from build123d import *
from build123d.topology import SkipClean

# Parameters (mm, degrees)
SKETCH1_W           = 100
SKETCH1_H           = 100
BOSS_EXTRUDE1_DEPTH = 100
CUT_EXTRUDE1_DEPTH  = 50
CIRPATTERN1_START   = -50
CIRPATTERN1_DEPTH   = 100
CIRPATTERN1_2_DEPTH = 50
SKETCH3_R           = 12.5
CUT_EXTRUDE2_DEPTH  = 22


with BuildPart() as part:
    # Sketch1 → Boss-Extrude1 (new body)
    with BuildSketch(Plane(origin=(0, 0, 0), x_dir=(1, 0, 0), z_dir=(0, 1, 0))):
        Rectangle(SKETCH1_W, SKETCH1_H)
    extrude(amount=BOSS_EXTRUDE1_DEPTH)

    # Sketch2 → Cut-Extrude1 (cut)
    with BuildSketch(Plane.ZY.offset(50)):
        with BuildLine():
            Line((0, 17.495781671), (-23.033292242, 50))
            ThreePointArc((-23.033292242, 50), (-11.516646121, 61.516646121), (0, 50))
            ThreePointArc((0, 50), (11.516646121, 61.516646121), (23.033292242, 50))
            Line((23.033292242, 50), (0, 17.495781671))
        make_face()
    extrude(amount=-CUT_EXTRUDE1_DEPTH, mode=Mode.SUBTRACT)

    # CirPattern1: read off the stored shape, not the designer's step
    # CirPattern1 outline → CirPattern1 (cut)
    with SkipClean():  # the faces are left unmerged after this step: merging them gives an invalid solid
        with BuildSketch(Plane.XY.offset(CIRPATTERN1_START)):
            with BuildLine():
                Line((-23.033292242, 50), (0, 17.495781671))
                Line((0, 17.495781671), (23.033292242, 50))
                ThreePointArc((23.033292242, 50), (11.516646121, 61.516646121), (0, 50))
                ThreePointArc((0, 50), (-11.516646121, 61.516646121), (-23.033292242, 50))
            make_face()
        extrude(amount=CIRPATTERN1_DEPTH, mode=Mode.SUBTRACT)

    # CirPattern1 2 outline → CirPattern1 2 (cut)
    with SkipClean():  # the faces are left unmerged after this step: merging them gives an invalid solid
        with BuildSketch(Plane.YZ):
            with BuildLine():
                Line((17.495781671, 0), (50, -23.033292242))
                ThreePointArc((50, -23.033292242), (61.516646121, -11.516646121), (50, 0))
                ThreePointArc((50, 0), (61.516646121, 11.516646121), (50, 23.033292242))
                Line((50, 23.033292242), (17.495781671, 0))
            make_face()
        extrude(amount=CIRPATTERN1_2_DEPTH, mode=Mode.SUBTRACT)

    # Sketch3 → Cut-Extrude2 (cut)
    with SkipClean():  # the faces are left unmerged after this step: merging them gives an invalid solid
        with BuildSketch(Plane(origin=(0, 100, 0), x_dir=(1, 0, 0), z_dir=(0, 1, 0))):
            with Locations(Location((0, 0, 0), (0, 0, 270))):
                Circle(SKETCH3_R)
        extrude(amount=-CUT_EXTRUDE2_DEPTH, mode=Mode.SUBTRACT)


solid = part.part
Source: CAD feature listing. Evaluate the final solid. Frame: model axes, mm. A direction names the side the tool comes from. Give positions to 0.01 mm unless a question says otherwise; leave off trailing zeros. Write each loop counter-clockwise with the first axis right and the second up, starting at its lowest first coordinate (ties: lowest second). Pieces come first, ordered by that corner, then holes. Notation, with made-up numbers: (-6.75, 54.5) -> (11.25, 54.5) arc R22 cw to (11.25, 74.5) -> close; hole circle Ø2 at (1.5, 9.5). An arc over 180 degrees is marked (long way). Write item = value, one per line.
Q1. Cut plane C-C on x = 7. Return loops of the section in (y, z).
Here are the results:
outline = (0, -50) -> (27.37, -50) -> (27.37, -7) -> (17.5, 0) -> (27.37, 7) -> (27.37, 50) -> (0, 50) -> close; (60.59, -50) -> (100, -50) -> (100, -10.36) -> (78, -10.36) -> (78, 10.36) -> (100, 10.36) -> (100, 50) -> (60.59, 50) -> (60.59, 16.03) arc R11.52 cw to (60.59, 7) -> (60.59, -7) arc R11.52 cw to (60.59, -16.03) -> close
Q2. Reachability of faces 1 (the face through (-35.304, 61.514, 11.263)), 2 (the face through (11.601, 61.516, -0.054)), 3 (the face through (-12, 100, -12)) from +Z, -Z, +X, -X, +Y, -Y: full face, straight path, thin tool, end or side. Return the list, or none.
Here are the results:
face_1 = +X, -X
face_2 = +Z, -Z
face_3 = +Z, -Z, +X, -X, +Y
Q3. Cut plane D-D on y = 30. Return loops of the section in (x, z), then the cut area to 3 significant figures.
Here are the results:
outline = (-50, -50) -> (-8.86, -50) -> (-8.86, -8.86) -> (-50, -8.86) -> close; (-50, 8.86) -> (-8.86, 8.86) -> (-8.86, 50) -> (-50, 50) -> close; (8.86, -50) -> (50, -50) -> (50, -8.86) -> (8.86, -8.86) -> close; (8.86, 8.86) -> (50, 8.86) -> (50, 50) -> (8.86, 50) -> close
area = 6,770 mm²
Q4. Cut plane B-B on x = 30.5. Return loops of the section in (y, z), then the cut area to 3 significant figures.
Here are the results:
outline = (0, -50) -> (100, -50) -> (100, 50) -> (0, 50) -> close; hole (17.5, 0) -> (50, -23.03) arc R11.52 ccw to (50, 0) arc R11.52 ccw to (50, 23.03) -> close
area = 8,830 mm²
Q5. Mould query, pull axis Y, two halves, no side actions, for faces 4 (the face through (50, 60, 1)), 5 (the face through (11.355, 33.52, 30.206)), 6 (the face through (0, 78, 0)). Classes: +Y half, -Y half, draft (parallel to the pull), parting line (faces both ways), or undercut.
Here are the results:
face_4 = draft
face_5 = undercut
face_6 = +Y half
Q6. Line query: line 1 (X direction, y = 83, z = 0); line 2 (X direction, y = 60.5, z = -17.5); line 3 (Z direction, x = 26.5, y = 43.5). Output: solid intervals per line, ascending. Write a range as from..to.
Here are the results:
line_1 = -50..-12.5, 12.5..50
line_2 = -50..-16.25, -6.79..6.79, 16.25..50
line_3 = -50..-18.43, 18.43..50
Q7. Cut plane A-A on z = 18. Return loops of the section in (x, y).
Here are the results:
outline = (-50, 0) -> (50, 0) -> (50, 42.9) -> (18, 42.9) -> (0, 17.5) -> (-18, 42.9) -> (-50, 42.9) -> close; (-50, 59.52) -> (-18, 59.52) arc R11.52 cw to (-5.03, 59.52) -> (5.03, 59.52) arc R11.52 cw to (18, 59.52) -> (50, 59.52) -> (50, 100) -> (-50, 100) -> close
